The listing builds one solid part. Answer for the finished solid, in the listing's coordinates (mm). A direction names the side the tool comes from. Give positions to 0.01 mm unless a question says otherwise; leave off trailing zeros. Order: outer loops, then holes, each group sorted by start corner. A loop starts at its lowest first (then second) coordinate and runs counter-clockwise, first axis right, second up. Notation, with made-up numbers: (-23, 52) - (22, 52) arc R28 ccw to (22, 82) - close; hole circle Ø1 at (20.5, 76.5). An arc over 180 degrees is marked (long way). Answer in a Markdown table with one row per item.
from build123d import *

# Parameters (mm, degrees)
BOSS_EXTRUDE1_DEPTH = 2.5
SKETCH4_R           = 1.24
BOSS_EXTRUDE2_DEPTH = 1.25
SKETCH5_R           = 1.25
CUT_EXTRUDE2_DEPTH  = 7.88
SKETCH7_R           = 1.875
CUT_EXTRUDE3_DEPTH  = 8.25
SKETCH8_R           = 1.875
BOSS_EXTRUDE3_DEPTH = 4.4
SKETCH5_3_R         = 1.25
CUT_EXTRUDE4_DEPTH  = 7.8800001


with BuildPart() as part:
    # Sketch3 → Boss-Extrude1 (new body, symmetric)
    with BuildSketch(Plane.XY):
        with BuildLine():
            Line((3.13, -2.065332903), (3.13, 2.065332903))
            ThreePointArc((3.13, 2.065332903), (-3.75, 0), (3.13, -2.065332903))
        make_face()
    extrude(amount=BOSS_EXTRUDE1_DEPTH, both=True)

    # Sketch4 → Boss-Extrude2 (add)
    with BuildSketch(Plane.XY.offset(2.5)):
        Circle(SKETCH4_R)
    boss_extrude2 = extrude(amount=BOSS_EXTRUDE2_DEPTH)

    # Mirror1: Boss-Extrude2 across plane
    add(boss_extrude2.mirror(Plane.XY))

    # Sketch5 → Cut-Extrude2 (cut, through all)
    with BuildSketch(Plane(origin=(3.13, 0, 0), x_dir=(0, 0, -1), z_dir=(1, 0, 0))):
        Circle(SKETCH5_R)
    extrude(amount=-CUT_EXTRUDE2_DEPTH, mode=Mode.SUBTRACT)

    # Sketch7 → Cut-Extrude3 (cut)
    with BuildSketch(Plane(origin=(3.13, 0, 0), x_dir=(0, 0, -1), z_dir=(1, 0, 0))):
        Circle(SKETCH7_R)
    extrude(amount=-CUT_EXTRUDE3_DEPTH, mode=Mode.SUBTRACT)

    # Sketch8 → Boss-Extrude3 (add)
    with BuildSketch(Plane(origin=(3.13, 0, 0), x_dir=(0, 0, -1), z_dir=(1, 0, 0))):
        Circle(SKETCH8_R)
    extrude(amount=-BOSS_EXTRUDE3_DEPTH)

    # Sketch5<3> → Cut-Extrude4 (cut, through all)
    with BuildSketch(Plane(origin=(3.13, 0, 0), x_dir=(0, 0, -1), z_dir=(1, 0, 0))):
        Circle(SKETCH5_3_R)
    extrude(amount=-CUT_EXTRUDE4_DEPTH, mode=Mode.SUBTRACT)


solid = part.part
Item 1: Find section B-B on x = 0. Write down the section's boundary in (y, z).
Answer block:
| item | result |
|---|---|
| outline | (-3.75, -2.5) - (-1.24, -2.5) - (-1.24, -3.75) - (1.24, -3.75) - (1.24, -2.5) - (3.75, -2.5) - (3.75, 2.5) - (1.24, 2.5) - (1.24, 3.75) - (-1.24, 3.75) - (-1.24, 2.5) - (-3.75, 2.5) - close; hole circle Ø2.5 at (0, 0) |
Item 2: Which of the six approach directions +Z, -Z, +X, -X, +Y, -Y give full straight-line access (tool end or side, diameter ignored) to faces 4 (the face through (0, 0, -3.75)), 5 (the face through (-2.49, 0.56, -1.79)), 6 (the face through (-3.086, 2.131, 0.035)), 7 (the face through (-0.27, -1.21, -3.12)), 8 (the face through (-1, 1, 2.5))?
Answer block:
| item | result |
|---|---|
| face 4 | -Z, +X, -X, +Y, -Y |
| face 5 | -X |
| face 6 | +Z, -Z |
| face 7 | -Z |
| face 8 | +Z |
Item 3: Find section A-A on y = 0. Write down the section's boundary in (x, z) (3 decimals).
Answer block:
| item | result |
|---|---|
| outline | (-3.75, -2.5) - (-1.24, -2.5) - (-1.24, -3.75) - (1.24, -3.75) - (1.24, -2.5) - (3.13, -2.5) - (3.13, -1.25) - (-1.27, -1.25) - (-1.27, -1.875) - (-3.75, -1.875) - close; (-3.75, 1.875) - (-1.27, 1.875) - (-1.27, 1.25) - (3.13, 1.25) - (3.13, 2.5) - (1.24, 2.5) - (1.24, 3.75) - (-1.24, 3.75) - (-1.24, 2.5) - (-3.75, 2.5) - close |
Item 4: Determine the mould class of faces 1 (the face through (-0.27, -1.21, 3.12)), 2 (the face through (0.96, -1.22, 0.27)), 3 (the face through (0, 0, 3.75)) for opening direction Y: pulls with the +Y half, pulls with the -Y half, needs draft (parallel to the pull), parting line crosses it, or undercut.
Answer block:
| item | result |
|---|---|
| face 1 | parting line crosses it |
| face 2 | undercut |
| face 3 | needs draft |
Item 5: Find section D-D on x = 2.25. Write down the section's boundary in (y, z), then the cut area to 3 significant figures.
Answer block:
| item | result |
|---|---|
| outline | (-3, -2.5) - (3, -2.5) - (3, 2.5) - (-3, 2.5) - close; hole circle Ø2.5 at (0, 0) |
| area | 25.1 mm² |
Item 6: Find section C-C on z = 0. Write down the section's boundary in (x, y) (3 decimals).
Answer block:
| item | result |
|---|---|
| outline | (-3.248, -1.875) arc R3.75 ccw to (3.13, -2.065) - (3.13, -1.25) - (-1.27, -1.25) - (-1.27, -1.875) - close; (-3.248, 1.875) - (-1.27, 1.875) - (-1.27, 1.25) - (3.13, 1.25) - (3.13, 2.065) arc R3.75 ccw to start |
Item 7: Consider line 1 (Z direction, x = -3.1, y = 0) (3 decimals); line 2 (Y direction, x = -0.75, z = -1); line 3 (X direction, y = -1.5, z = 1). Determine where each line is inside the solid, lowest interval first.
Answer block:
| item | result |
|---|---|
| line 1 | -2.5 to -1.875, 1.875 to 2.5 |
| line 2 | -3.67 to -0.75, 0.75 to 3.67 |
| line 3 | -1.27 to 3.13 |
Item 8: Each of these flat-tipped pins is pushed along its axis until it touches: P1, Ø1, axis at x = -3, z = 2, coming from the -Y side; P2, Ø2, axis at x = 2, z = 2.5, coming from the -Y side. Where does it stop, or does it pass through?
Answer block:
| item | result |
|---|---|
| P1 | y = -2.8 |
| P2 | y = -3.61 |
